from build123d import *

# Parameters (mm, degrees)
F0_W     = 27.5
F0_H     = 27.4
F1_DEPTH = 1.22
F2_W     = 14.1
F2_H     = 2.3066
F3_DEPTH = 25.4
F4_W     = 27.1
F4_H     = 14.88
F5_DEPTH = 1.57
F7_D     = 1.85
F8_W     = 17.84
F8_H     = 2.3
F9_DEPTH = 11.28


with BuildPart() as f1:
    # F0 (on Top) → F1 (new body)
    with BuildSketch(Plane.XY):
        Rectangle(F0_W, F0_H)
    extrude(amount=F1_DEPTH)

    # F2 (on face) → F3 (cut)
    with BuildSketch(Plane.XY.offset(1.22)):
        with Locations((0, -12.5467)):
            Rectangle(F2_W, F2_H)
    extrude(amount=-F3_DEPTH, mode=Mode.SUBTRACT)

    # F4 (on face) → F5 (join)
    with BuildSketch(Plane.XY.offset(1.22)):
        with Locations((0, 1.74)):
            Rectangle(F4_W, F4_H)
    extrude(amount=F5_DEPTH)

    # F7 (through all)
    with Locations(Plane.XY.offset(1.22)):
        with Locations((-11.9, -11.85), (-11.9, 11.85), (11.9, 11.85), (11.9, -11.85)):
            Hole(F7_D / 2)

    # F8 (on face) → F9 (join)
    with BuildSketch(Plane(origin=(0, 0, 0), x_dir=(1, 0, 0), z_dir=(0, 0, -1))):
        with Locations((0, -12.55)):
            Rectangle(F8_W, F8_H)
    extrude(amount=F9_DEPTH)


solid = f1.part
Geometry check sheet. Reference: the model listing, model coordinates, mm. A direction names the side the tool comes from. Coordinates: 2 decimals unless noted, no trailing zeros. Order: outer loops, then holes, each group sorted by start corner. A loop starts at its lowest first (then second) coordinate and runs counter-clockwise, first axis right, second up. Notation, with made-up numbers: (-33.75, -40) -> (-7.75, -40) arc R6 ccw to (-7.75, -33) -> close; hole circle Ø6 at (53.5, -7). An arc over 180 degrees is marked (long way). Use a Markdown table: item, result. Add a question column.
1. Cross-section at D-D (x = 0.5). Enter the section's corners in (y, z).
2. Cross-section at B-B (x = 11.9). Enter the section's corners in (y, z) (3 decimals).
3. Material ranges on L1, parallel to Y at x = 11.9, z = 0.6 (3 decimals); L2, parallel to Z at x = 8.25, y = 12; L3, parallel to Y at x = 6.5, z = -1.75, recorded low to high.
4. Cross-section at C-C (y = 11.85). Enter the section's corners in (x, z) (3 decimals), and give its area (3 significant figures).
5. Mould release check, pull along X, two halves, no side actions. Record for faces 1 (the face through (0, 9.18, 2)), 2 (the face through (-8.92, 13, -6)), 3 (the face through (-12.754, 11.496, 0.601)): pulls with the +X half, pulls with the -X half, needs draft (parallel to the pull), parting line crosses it, or undercut.
6. Go/stop test with flat-tipped pins: pin 1 Ø1.3 at (y, z) = (3, 2) entering from +X; pin 2 Ø5 at (y, z) = (-5, -3) entering from -X; pin 3 Ø1.3 at (x, z) = (-1.5, 2) entering from +Y; pin 4 Ø1.3 at (x, z) = (-3, 1) entering from -Y. Record where each tip stops, or that it passes through.
7. Set-up check for faces 4 (the face through (0, 11.4, -6)), 5 (the face through (-7.05, -13, 1)), 6 (the face through (13.55, 2, 2)): record each of +Z, -Z, +X, -X, +Y, -Y from which the full face is reachable in a straight line by a thin tool's end or side.
8. Cross-section at A-A (y = -11.85). Enter the section's corners in (x, z) (3 decimals), and give its area (3 significant figures).
Filled sheet:
| question | item | result |
|---|---|---|
| 1 | outline | (-11.39, 0) -> (11.4, 0) -> (11.4, -11.28) -> (13.7, -11.28) -> (13.7, 1.22) -> (9.18, 1.22) -> (9.18, 2.79) -> (-5.7, 2.79) -> (-5.7, 1.22) -> (-11.39, 1.22) -> close |
| 2 | outline | (-13.7, 0) -> (-12.775, 0) -> (-12.775, 1.22) -> (-13.7, 1.22) -> close; (-10.925, 0) -> (10.925, 0) -> (10.925, 1.22) -> (9.18, 1.22) -> (9.18, 2.79) -> (-5.7, 2.79) -> (-5.7, 1.22) -> (-10.925, 1.22) -> close; (12.775, 0) -> (13.7, 0) -> (13.7, 1.22) -> (12.775, 1.22) -> close |
| 3 | L1 | -13.7 to -12.775, -10.925 to 10.925, 12.775 to 13.7 |
| 3 | L2 | -11.28 to 1.22 |
| 3 | L3 | 11.4 to 13.7 |
| 4 | outline | (-13.75, 0) -> (-12.825, 0) -> (-12.825, 1.22) -> (-13.75, 1.22) -> close; (-10.975, 0) -> (-8.92, 0) -> (-8.92, -11.28) -> (8.92, -11.28) -> (8.92, 0) -> (10.975, 0) -> (10.975, 1.22) -> (-10.975, 1.22) -> close; (12.825, 0) -> (13.75, 0) -> (13.75, 1.22) -> (12.825, 1.22) -> close |
| 4 | area | 230 mm2 |
| 5 | face 1 | needs draft |
| 5 | face 2 | pulls with the -X half |
| 5 | face 3 | undercut |
| 6 | pin 1 | x = 13.55 |
| 6 | pin 2 | through |
| 6 | pin 3 | y = 9.18 |
| 6 | pin 4 | y = -11.39 |
| 7 | face 4 | -Z, +X, -X, -Y |
| 7 | face 5 | +Z, -Z, -Y |
| 7 | face 6 | +Z, +X, +Y, -Y |
| 8 | outline | (-13.75, 0) -> (-12.825, 0) -> (-12.825, 1.22) -> (-13.75, 1.22) -> close; (-10.975, 0) -> (-7.05, 0) -> (-7.05, 1.22) -> (-10.975, 1.22) -> close; (7.05, 0) -> (10.975, 0) -> (10.975, 1.22) -> (7.05, 1.22) -> close; (12.825, 0) -> (13.75, 0) -> (13.75, 1.22) -> (12.825, 1.22) -> close |
| 8 | area | 11.8 mm2 |
